```python
from build123d import *

# Parameters (mm, degrees)
SKETCH1_W = 4
SKETCH1_H = 8


# Read off the part's stored shape, not the designer's step: Shell1
with BuildPart() as part:
    # Sketch1 → Revolve1 (revolve)
    with BuildSketch(Plane.YZ, mode=Mode.PRIVATE) as revolve1_sk:
        with BuildLine():
            Line((0, 13), (0, 9))
            Line((0, 9), (4, 9))
            ThreePointArc((4, 9), (2.828427125, 11.828427125), (0, 13))
        make_face()
        with Locations((2, 5)):
            Rectangle(SKETCH1_W, SKETCH1_H)
        Polygon((4, 1), (0, 1), (0, 0), (4.5, 0), (4.5, 1), align=None)
    revolve(revolve1_sk.sketch.rotate(Axis((0, 0, 10.805456946), (0, 0, -1)), 90), axis=Axis((0, 0, 10.805456946), (0, 0, -1)))

    # Shell1 outline → Shell1 (revolve, cut)
    with BuildSketch(Plane.XZ):
        with BuildLine():
            Line((0, 0), (3, 0))
            Line((3, 0), (3, 8.999999997))
            ThreePointArc((3, 8.999999997), (2.121320345, 11.121320342), (0, 12))
            Line((0, 12), (0, 0))
        make_face()
    revolve(axis=Axis((0, 0, 0), (0, 0, 1)), mode=Mode.SUBTRACT)


solid = part.part
```
Geometry check sheet. Reference: the model listing, model coordinates, mm. A direction names the side the tool comes from. Coordinates: 2 decimals unless noted, no trailing zeros. Write each loop counter-clockwise with the first axis right and the second up, starting at its lowest first coordinate (ties: lowest second). Pieces come first, ordered by that corner, then holes. Notation, with made-up numbers: M 88,-39 L 99,-39 A19 cw 99,-27 Z; hole C 73,-8.5 d10. An arc over 180 degrees is marked long. One line per item, written item: value. Start each with the question number.
(1) Depth check by flat-ended pin: pin 1 (2.5 mm diameter, centred on x = 2, y = -1, fed in from +Z); pin 2 (1 mm diameter, centred on x = -2, z = 11, fed in from -Y); pin 3 (5 mm diameter, centred on x = -1, z = 11, fed in from -Y). Enter the tip coordinate at first touch or a pass-through.
(2) Tool access check on faces 4 (the face through (-3.32, -3.04, 0.51)), 5 (the face through (-3, 3, 1)). Record the directions out of +Z, -Z, +X, -X, +Y, -Y that give a thin tool (end or side, any length) a straight path to the whole face; none if there is none.
(3) Sectioned sample at A-A, the plane y = 0. Enter the section's corners in (x, z), and give its area (3 significant figures).
(4) Release check for a two-part mould opening along Y. For faces 1 (the face through (-0.867, 3.905, 5.056)), 2 (the face through (-1, 3, 0)), 3 (the face through (-3, 0, 5)) record: released by +Y, released by -Y, zero draft, split by the parting line, or undercut.
(5) Sectioned sample at C-C, the plane z = 12.25. Enter the section's corners in (x, y).
(6) Scan lines: line 1 along Y through (x, z) = (0, 2.75); line 2 along Y through (x, z) = (1.75, 8.25); line 3 along X through (y, z) = (-2, 6.75). Record each from-to range of solid material in increasing order. Write a range as [from, to].
(7) Sectioned sample at D-D, the plane y = -1.75. Enter the section's corners in (x, z).
Filled sheet:
1. pin 1: z = 12.88
1. pin 2: y = -3.25
1. pin 3: y = -4
2. face 4: +Z, -Z
2. face 5: +Z
3. outline: M -4.5,0 L -3,0 L -3,9 A3 cw 3,9 L 3,0 L 4.5,0 L 4.5,1 L 4,1 L 4,9 A4 ccw -4,9 L -4,1 L -4.5,1 Z
3. area: 30.0 mm²
4. face 1: split by the parting line
4. face 2: zero draft
4. face 3: undercut
5. outline: C 0,0 d4.66
6. line 1: [-4, -3], [3, 4]
6. line 2: [-3.6, -2.44], [2.44, 3.6]
6. line 3: [-3.46, -2.24], [2.24, 3.46]
7. outline: M -4.15,0 L -2.44,0 L -2.44,9 A2.44 cw 2.44,9 L 2.44,0 L 4.15,0 L 4.15,1 L 3.6,1 L 3.6,9 A3.6 ccw -3.6,9 L -3.6,1 L -4.15,1 Z
